from build123d import *

# Parameters (mm, degrees)
F0_W      = 50.8
F0_H      = 86.36
F1_DEPTH  = 63.5
F2_W      = 20.32
F2_H      = 43.18
F2_W_2    = 17.78
F2_H_2    = 12.7
F3_DEPTH  = 228.6
F5_DEPTH  = 228.6
F6_W      = 86.36
F6_H      = 50.8
F6_H_2    = 63.5
F7_DEPTH  = 127
F9_W      = 127
F9_H      = 50.8
F10_DEPTH = 228.6
F12_DEPTH = 37.999924
F13_DEPTH = 86.36
F15_DEPTH = 101.6
F16_W     = 41.91
F16_H     = 22.225
F17_DEPTH = 228.6
F18_W     = 46.355
F18_H     = 86.36
F18_W_2   = 4.445
F19_DEPTH = 12.7
F20_W     = 12.7
F20_H     = 9.525
F20_W_2   = 3.175
F20_W_3   = 6.35
F20_H_2   = 3.175
F21_DEPTH = 228.6
F23_DEPTH = 228.6
F25_DEPTH = 59.69


with BuildPart() as f1:
    # F0 (on Top) → F1 (new body)
    with BuildSketch(Plane.XY):
        with Locations((0, 4.4812522829)):
            Rectangle(F0_W, F0_H)
    extrude(amount=F1_DEPTH)

    # F2 (on face) → F3 (cut)
    with BuildSketch(Plane.XY.offset(63.5)):
        with Locations((10.16, -17.1087477171)):
            Rectangle(F2_W, F2_H)
        with Locations((-8.89, -17.1087477171)):
            Rectangle(F2_W_2, F2_H)
        with Locations((-8.89, 10.8312522829)):
            Rectangle(F2_W_2, F2_H_2)
        with Locations((10.16, 10.8312522829)):
            Rectangle(F2_W, F2_H_2)
    extrude(amount=-F3_DEPTH, mode=Mode.SUBTRACT)

    # F4 (on face) → F5 (cut)
    with BuildSketch(Plane(origin=(0, 47.6612522829, 0), x_dir=(-1, 0, 0), z_dir=(0, 1, 0))):
        Polygon((-25.4, 63.5), (25.4, 31.75), (25.4, 63.5), align=None)
    extrude(amount=-F5_DEPTH, mode=Mode.SUBTRACT)

    # F6 (on face) → F7 (join)
    with BuildSketch(Plane.YZ.offset(25.4)):
        with Locations((4.4812522829, 88.9)):
            Rectangle(F6_W, F6_H)
        with Locations((4.4812522829, 31.75)):
            Rectangle(F6_W, F6_H_2)
    extrude(amount=F7_DEPTH)

    # F9 (on face) → F10 (cut)
    with BuildSketch(Plane.XZ.offset(38.6987477171)):
        with Locations((88.9, 88.9)):
            Rectangle(F9_W, F9_H)
    extrude(amount=-F10_DEPTH, mode=Mode.SUBTRACT)

    # F11 (on face) → F12 (cut)
    with BuildSketch(Plane.XZ.offset(38.6987477171)):
        Polygon((107.95, 5.08), (107.95, 13.3552532643), (107.95, 25.18000044), (67.1500054, 25.18000044), (67.1500054, 5.08), align=None)
    extrude(amount=-F12_DEPTH, mode=Mode.SUBTRACT)

    # F8 (on face) → F13 (join)
    with BuildSketch(Plane.XZ.offset(38.6987477171)):
        with BuildLine():
            Line((59.7608433873, 63.5), (101.6, 63.5))
            Line((101.6, 63.5), (101.6, 88.9))
            add(Edge.make_bspline(
                [(101.6, 88.9), (79.3954620772, 84.9506698417), (69.3900678517, 65.6088911006), (59.7608433873, 63.5)],
                knots=[0, 0, 0, 0, 0.338800951, 0.338800951, 0.338800951, 0.338800951], degree=3))
        make_face()
        Polygon((101.6, 88.9), (101.6, 63.5), (152.4, 63.5), (152.4, 114.3), (101.6, 114.3), align=None)
    extrude(amount=-F13_DEPTH)

    # F14 (on face) → F15 (cut)
    with BuildSketch(Plane.YZ.offset(152.4)):
        Polygon((47.6612522829, 114.3), (-38.6987477171, 114.3), (-38.6987477171, 88.9), (47.6612522829, 88.9), (47.6612522829, 101.6), align=None)
    extrude(amount=-F15_DEPTH, mode=Mode.SUBTRACT)

    # F16 (on face) → F17 (cut)
    with BuildSketch(Plane.XZ.offset(38.6987477171)):
        with BuildLine():
            Line((110.49, 88.9), (106.045, 88.9))
            add(Edge.make_bspline(
                [(106.045, 88.9), (105.9615328839, 79.9996478624), (106.6244970851, 72.6786467547), (107.8523208869, 66.675)],
                knots=[0, 0, 0, 0, 0.1081078186, 0.1081078186, 0.1081078186, 0.1081078186], degree=3))
            Line((107.8523208869, 66.675), (110.49, 66.675))
            Line((110.49, 66.675), (110.49, 88.9))
        make_face()
        with Locations((131.445, 77.7875)):
            Rectangle(F16_W, F16_H)
        with BuildLine():
            add(Edge.make_bspline(
                [(125.4735723701, 42.0280762083), (135.9858471133, 38.600025516), (147.748179628, 43.4285939835), (152.4, 44.45)],
                knots=[0.3864894569, 0.3864894569, 0.3864894569, 0.3864894569, 0.7739727648, 0.7739727648, 0.7739727648, 0.7739727648], degree=3))
            Line((125.4735723701, 42.0280762083), (125.4735723701, 0))
            Line((125.4735723701, 0), (152.4, 0))
            Line((152.4, 0), (152.4, 44.45))
        make_face()
        with BuildLine():
            Line((152.4, 66.675), (110.49, 66.675))
            Line((110.49, 66.675), (110.49, 57.590838654))
            add(Edge.make_bspline(
                [(110.49, 57.590838654), (114.1247988782, 48.4297517127), (119.6043502671, 43.9420283629), (125.4735723701, 42.0280762083)],
                knots=[0.1701494495, 0.1701494495, 0.1701494495, 0.1701494495, 0.3864894569, 0.3864894569, 0.3864894569, 0.3864894569], degree=3))
            add(Edge.make_bspline(
                [(125.4735723701, 42.0280762083), (135.9858471133, 38.600025516), (147.748179628, 43.4285939835), (152.4, 44.45)],
                knots=[0.3864894569, 0.3864894569, 0.3864894569, 0.3864894569, 0.7739727648, 0.7739727648, 0.7739727648, 0.7739727648], degree=3))
            Line((152.4, 44.45), (152.4, 66.675))
        make_face()
        with BuildLine():
            Line((110.49, 66.675), (107.8523208869, 66.675))
            add(Edge.make_bspline(
                [(107.8523208869, 66.675), (108.556952542, 63.2295874388), (109.4476183658, 60.2180400746), (110.49, 57.590838654)],
                knots=[0.1081078186, 0.1081078186, 0.1081078186, 0.1081078186, 0.1701494495, 0.1701494495, 0.1701494495, 0.1701494495], degree=3))
            Line((110.49, 57.590838654), (110.49, 66.675))
        make_face()
    extrude(amount=-F17_DEPTH, mode=Mode.SUBTRACT)

    # F18 (on face) → F19 (join)
    with BuildSketch(Plane.XY.offset(88.9)):
        with Locations((129.2225, 4.4812522829)):
            Rectangle(F18_W, F18_H)
        with Locations((103.8225, 4.4812522829)):
            Rectangle(F18_W_2, F18_H)
    extrude(amount=F19_DEPTH)

    # F20 (on face) → F21 (cut)
    with BuildSketch(Plane.XZ.offset(38.6987477171)):
        with Locations((107.95, 96.8375)):
            Rectangle(F20_W, F20_H)
        Polygon((127, 99.695), (127, 101.6), (114.3, 101.6), (114.3, 92.075), align=None)
        Polygon((127, 99.695), (130.175, 101.6), (127, 101.6), align=None)
        with Locations((131.7625, 96.8375)):
            Rectangle(F20_W_2, F20_H)
        with Locations((136.525, 96.8375)):
            Rectangle(F20_W_3, F20_H)
        with Locations((131.7625, 90.4875)):
            Rectangle(F20_W_2, F20_H_2)
        with Locations((136.525, 90.4875)):
            Rectangle(F20_W_3, F20_H_2)
        Polygon((152.4, 95.25), (152.4, 101.6), (139.7, 101.6), (139.7, 92.075), (152.4, 92.075), align=None)
        with Locations((146.05, 90.4875)):
            Rectangle(F20_W, F20_H_2)
    extrude(amount=-F21_DEPTH, mode=Mode.SUBTRACT)

    # F22 (on face) → F23 (cut)
    with BuildSketch(Plane.XZ.offset(38.6987477171)):
        Polygon((122.2375, 92.075), (114.3, 88.9), (130.175, 88.9), align=None)
    extrude(amount=-F23_DEPTH, mode=Mode.SUBTRACT)

    # F24 (on face) → F25 (cut)
    with BuildSketch(Plane(origin=(107.95, 0, 0), x_dir=(0, -1, 0), z_dir=(-1, 0, 0))):
        Polygon((22.0737809671, 5.08), (22.2987805171, 5.08), (22.2987805171, 10.2799896), (17.0987909171, 10.2799896), (17.0987909171, 5.08), (17.3237904671, 5.08), (19.6987857171, 5.08), align=None)
    extrude(amount=-F25_DEPTH, mode=Mode.SUBTRACT)


solid = f1.part
The model under review builds one solid part; all positions refer to its coordinate system, in mm. A direction names the side the tool comes from. Coordinates: 2 decimals unless noted, no trailing zeros. Loops run counter-clockwise (first coordinate to the right, second up) from the corner with the lowest first, then second, coordinate; pieces in that order, holes last.
(1) Tool access review of faces 4 (the flat face through (110, 5, 88.9)), 5 (the flat face through (101.6, 4, 90)), 6 (the flat face through (118.3, 3.9, 90.5)), 7 (the flat face through (2, 17.181, 24)): name each direction out of +Z, -Z, +X, -X, +Y, -Y from which nothing blocks a thin tool from reaching the whole face with its end or side.
Determined:
face 4: +X, +Y, -Y
face 5: +Z, -X, +Y, -Y
face 6: +Y, -Y
face 7: +Z, -Z, -Y
(2) Draft analysis for pull direction Y (two halves, no side actions). For faces 1 (the flat face through (108, 4, 92.075)), 2 (the flat face through (74, -38.699, 39)), 3 (the flat face through (117, -20, 10.28)), state which applies: +Y half, -Y half, draft (parallel to the pull), parting line (faces both ways), or undercut.
Determined:
face 1: draft
face 2: -Y half
face 3: undercut
(3) Consider section C-C, the plane x = 55. Give the boundary of the cut face in (y, z), plus the area to 3 significant figures.
Determined:
outline: (-38.7, 0) - (47.66, 0) - (47.66, 63.5) - (-38.7, 63.5) - close
area: 5,480 mm2
(4) Consider section D-D, the plane z = 94.5. Give the boundary of the cut face in (x, y) (3 decimals), plus the area to 3 significant figures.
Determined:
outline: (118.342, -38.699) - (130.175, -38.699) - (130.175, 47.661) - (118.342, 47.661) - close
area: 1,020 mm2
(5) Consider section B-B, the plane y = -15. Give the number of separate pieces and of enclosed holes in the cut face, plus the area to 3 significant figures.
Determined:
separate pieces: 2
enclosed holes: 1
area: 6,740 mm2
(6) Consider section A-A, the plane z = 13. Give the boundary of the cut face in (x, y), plus the area to 3 significant figures.
Determined:
outline: (-25.4, -38.7) - (-17.78, -38.7) - (-17.78, 17.18) - (20.32, 17.18) - (20.32, -38.7) - (67.15, -38.7) - (67.15, -0.7) - (107.95, -0.7) - (107.95, -38.7) - (125.47, -38.7) - (125.47, 47.66) - (-25.4, 47.66) - close
area: 9,350 mm2
(7) Insertion check: P1, Ø4, axis at x = 109, y = 24.5, coming from the +Z side (3 decimals); P2, Ø4, axis at x = 16, z = 15.5, coming from the -Y side; P3, Ø1.6, axis at y = -16, z = 90.5, coming from the -X side; P4, Ø1.5, axis at x = 95, y = -26.5, coming from the -Z side. Each pin has a flat end and moves straight along its axis. Give the tip position at first contact, or say it passes through.
Determined:
P1: stops at z = 92.075
P2: stops at y = 17.18
P3: stops at x = 101.6
P4: stops at z = 0
(8) Wall thickness on L1, parallel to X at y = 7.5, z = 22; L2, parallel to Z at x = 29, y = -23; L3, parallel to Z at x = 113.5, y = -23 (3 decimals): over which ranges is each line inside the solid? List them lowest first.
Determined:
L1: x = -25.4 to -17.78, 20.32 to 125.47
L2: z = 0 to 63.5
L3: z = 0 to 51.625, 88.9 to 92.075
